Could you check a few things on this drawing? It's one solid part, dimensions in mm from its lowest x, y, z. Round coordinates to 2 decimals unless told otherwise and drop trailing zeros. Loops run counter-clockwise (first coordinate to the right, second up) from the corner with the lowest first, then second, coordinate; pieces in that order, holes last.
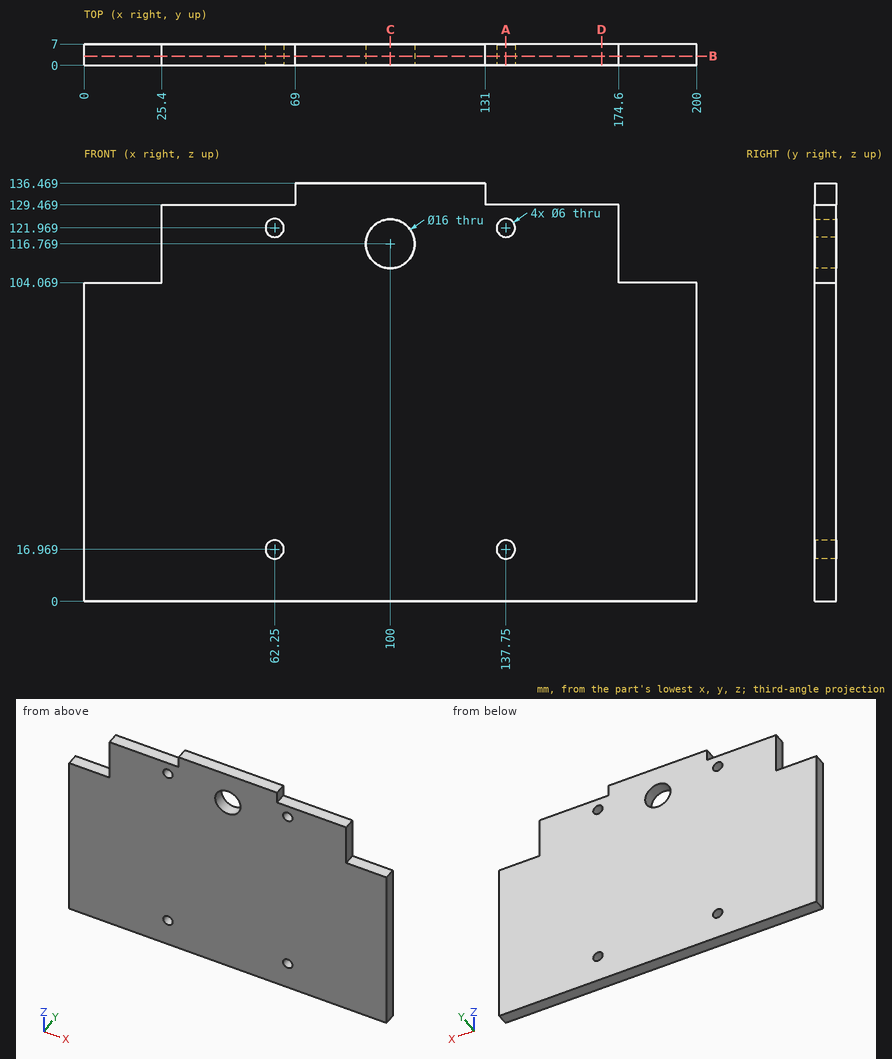
(1) For pin 1 (2 mm diameter, centred on x = 17.5, y = 3.5, fed in from +Z); pin 2 (2 mm diameter, centred on x = 55, y = 4, fed in from +Z); pin 3 (3.5 mm diameter, centred on y = 5, z = 112, fed in from -X), each with a flat end and sliding along its axis, tell me the tip position at first contact or that it passes through.
(2) Suppose I cut it at D-D (x = 169). Write out the boundary of the cut face in (y, z).
(3) If I drill on line 1 (Z direction, x = 138, y = 1.25); line 2 (X direction, y = 6.25, z = 18); line 3 (Z direction, x = 100, y = 2.75), over which ranges is the centre line in solid material (lowest first)?
(4) Suppose I cut it at A-A (x = 137.75). Write out the boundary of the cut face in (y, z).
(5) Suppose I cut it at C-C (x = 100). Write out the boundary of the cut face in (y, z).
(6) Suppose I cut it at B-B (y = 3). Write out the boundary of the cut face in (x, z), then the cut area to 3 significant figures.
Check result:
1. pin 1: stops at z = 104.07
1. pin 2: stops at z = 129.47
1. pin 3: stops at x = 25.4
2. outline: (0, 0) - (7, 0) - (7, 129.47) - (0, 129.47) - close
3. line 1: z = 0 to 13.98, 19.96 to 118.98, 124.96 to 129.47
3. line 2: x = 0 to 59.43, 65.07 to 134.93, 140.57 to 200
3. line 3: z = 0 to 108.77, 124.77 to 136.47
4. outline: (0, 0) - (7, 0) - (7, 13.97) - (0, 13.97) - close; (0, 19.97) - (7, 19.97) - (7, 118.97) - (0, 118.97) - close; (0, 124.97) - (7, 124.97) - (7, 129.47) - (0, 129.47) - close
5. outline: (0, 0) - (7, 0) - (7, 108.77) - (0, 108.77) - close; (0, 124.77) - (7, 124.77) - (7, 136.47) - (0, 136.47) - close
6. outline: (0, 0) - (200, 0) - (200, 104.07) - (174.6, 104.07) - (174.6, 129.47) - (131, 129.47) - (131, 136.47) - (69, 136.47) - (69, 129.47) - (25.4, 129.47) - (25.4, 104.07) - (0, 104.07) - close; hole circle Ø6 at (62.25, 16.97); hole circle Ø6 at (62.25, 121.97); hole circle Ø16 at (100, 116.77); hole circle Ø6 at (137.75, 16.97); hole circle Ø6 at (137.75, 121.97)
6. area: 24,700 mm2
